The figure shows three views and two pictorial views of one solid part (mm, origin at its lowest corner). Answer the questions. Round coordinates to 2 decimals unless told otherwise and drop trailing zeros. Loops run counter-clockwise (first coordinate to the right, second up) from the corner with the lowest first, then second, coordinate; pieces in that order, holes last. Notation, with made-up numbers: (-18, 51.5) -> (15, 51.5) arc R27 ccw to (15, 74.5) -> close; hole circle Ø5 at (-7.5, 0). An arc over 180 degrees is marked (long way). Write each question's results on one line, items separated by ' | '. Start each with the question number.
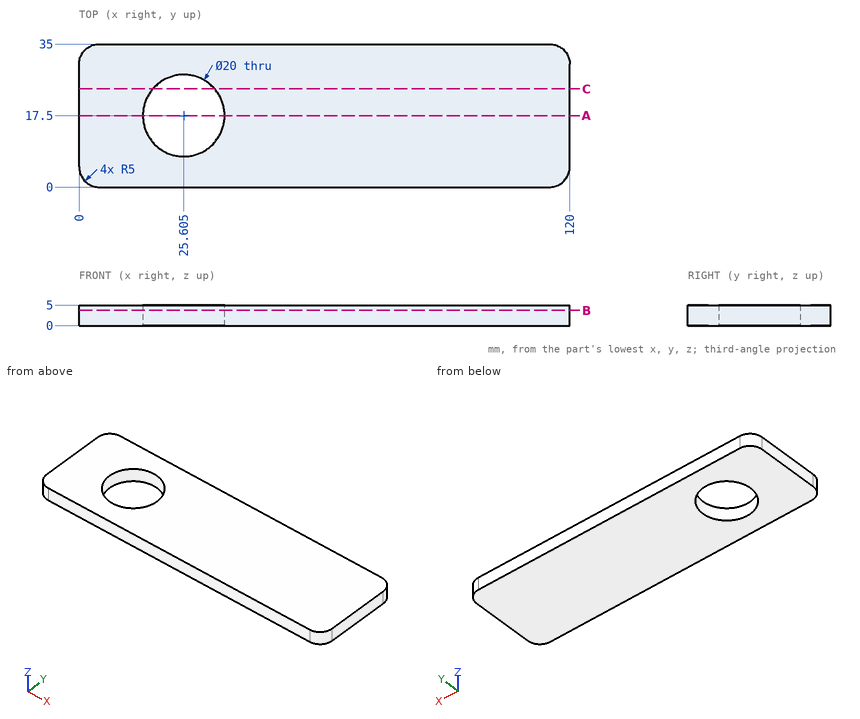
Item 1: The part is cut by section B-B, the plane z = 3.75. Give the vertices of the cut face in (x, y) (1 decimal), plus the area to 3 significant figures.
Item 2: The part is cut by section A-A, the plane y = 17.5. Give the vertices of the cut face in (x, z) (1 decimal), plus the area to 3 significant figures.
Item 3: The part is cut by section C-C, the plane y = 24. Give the vertices of the cut face in (x, z) (1 decimal).
Item 4: Straight lines are drawn through the part: L1, parallel to Y at x = 27.5, z = 1.35; L2, parallel to X at y = 15, z = 3.4; L3, parallel to Y at x = 29.5, z = 2.1. For each, find the intervals that lie inside material, in ascending order. Write a range as [from, to].
Report:
1) outline: (0, 5) arc R5 ccw to (5, 0) -> (115, 0) arc R5 ccw to (120, 5) -> (120, 30) arc R5 ccw to (115, 35) -> (5, 35) arc R5 ccw to (0, 30) -> close; hole circle Ø20 at (25.6, 17.5) | area: 3,860 mm2
2) outline: (0, 0) -> (15.6, 0) -> (15.6, 5) -> (0, 5) -> close; (35.6, 0) -> (120, 0) -> (120, 5) -> (35.6, 5) -> close | area: 500 mm2
3) outline: (0, 0) -> (18, 0) -> (18, 5) -> (0, 5) -> close; (33.2, 0) -> (120, 0) -> (120, 5) -> (33.2, 5) -> close
4) L1: y = [0, 7.68], [27.32, 35] | L2: x = [0, 15.92], [35.29, 120] | L3: y = [0, 8.29], [26.71, 35]
